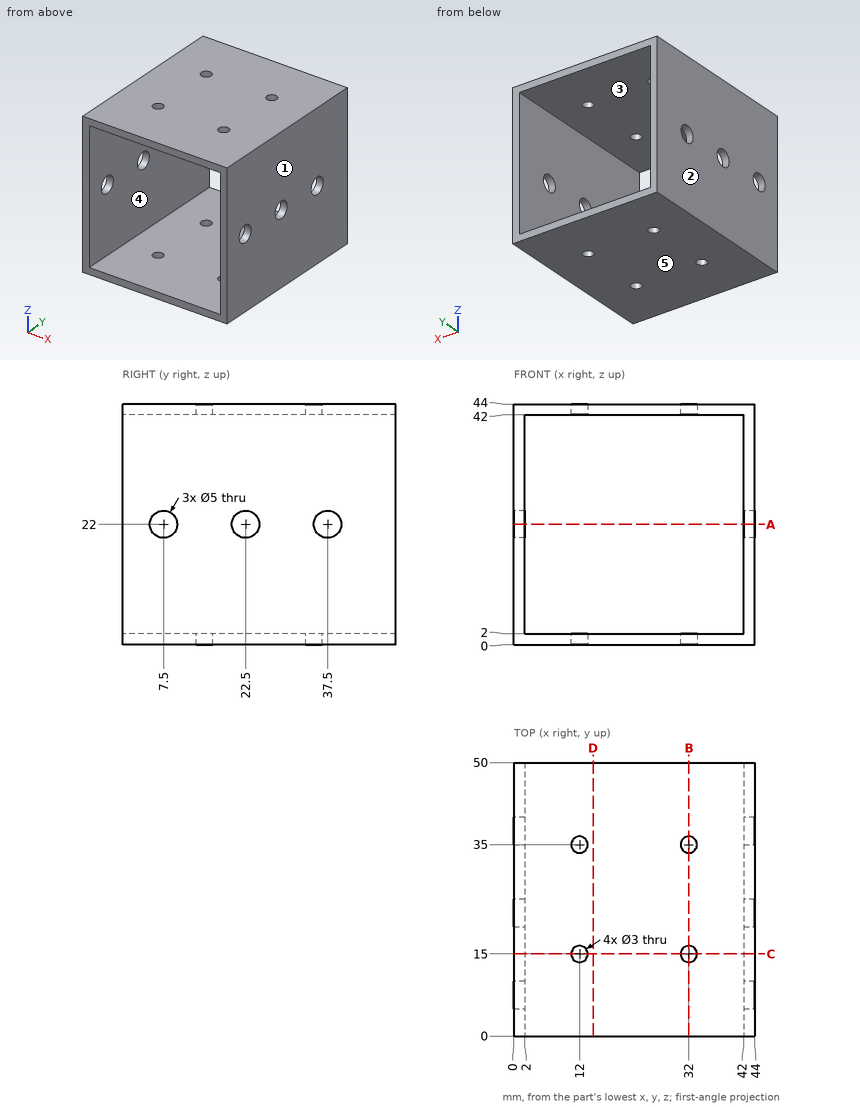
Geometry: see drawing. Coordinates: mm, zero at the bounding-box minimum. A direction names the side the tool comes from. Coordinates: 2 decimals unless noted, no trailing zeros. Loops run counter-clockwise (first coordinate to the right, second up) from the corner with the lowest first, then second, coordinate; pieces in that order, holes last. Notation, with made-up numbers: (17, 43.25) - (28, 43.25) arc R20 ccw to (28, 77.25) - close; hole circle Ø3 at (-14.75, 61). An arc over 180 degrees is marked (long way). Return JSON: item names as keys, results as strings.
Q1. Contact query for a flat-ended pin moving along its axis: P1, Ø3, axis at y = 7.5, z = 22, coming from the +X side. Output: stop coordinate, or through.
Results:
{"P1": "through"}
Q2. Section B-B, the plane x = 32. Return loops of the section in (y, z), plus the area to 3 significant figures.
Results:
{"outline": "(0, 0) - (13.5, 0) - (13.5, 2) - (0, 2) - close; (0, 42) - (13.5, 42) - (13.5, 44) - (0, 44) - close; (16.5, 0) - (33.5, 0) - (33.5, 2) - (16.5, 2) - close; (16.5, 42) - (33.5, 42) - (33.5, 44) - (16.5, 44) - close; (36.5, 0) - (50, 0) - (50, 2) - (36.5, 2) - close; (36.5, 42) - (50, 42) - (50, 44) - (36.5, 44) - close", "area": "176 mm2"}
Q3. Section A-A, the plane z = 22. Give the number of separate pieces and of enclosed holes in the cut face, plus the area to 3 significant figures.
Results:
{"separate pieces": "8", "enclosed holes": "0", "area": "140 mm2"}
Q4. Section D-D, the plane x = 14.5. Return loops of the section in (y, z).
Results:
{"outline": "(0, 0) - (50, 0) - (50, 2) - (0, 2) - close; (0, 42) - (50, 42) - (50, 44) - (0, 44) - close"}
Q5. Section C-C, the plane y = 15. Return loops of the section in (x, z), plus the area to 3 significant figures.
Results:
{"outline": "(0, 0) - (10.5, 0) - (10.5, 2) - (2, 2) - (2, 42) - (10.5, 42) - (10.5, 44) - (0, 44) - close; (13.5, 0) - (30.5, 0) - (30.5, 2) - (13.5, 2) - close; (13.5, 42) - (30.5, 42) - (30.5, 44) - (13.5, 44) - close; (33.5, 0) - (44, 0) - (44, 44) - (33.5, 44) - (33.5, 42) - (42, 42) - (42, 2) - (33.5, 2) - close", "area": "312 mm2"}
Q6. Mould query, pull axis X, two halves, no side actions, for the marked faces 1, 2 and 3. Classes: released by +X, released by -X, zero draft, split by the parting line, or undercut.
Results:
{"face 1": "released by +X", "face 2": "released by -X", "face 3": "undercut"}
Q7. Access query for the marked faces 4 and 5. Directions: +Z, -Z, +X, -X, +Y, -Y. A direction counts if a zero-diameter tool reaches every point of the face in a straight line with its end or side. Return the directions, or none.
Results:
{"face 4": "+Y, -Y", "face 5": "-Z, +X, -X, +Y, -Y"}
Q8. Material intervals for line 1 along Y through (x, z) = (12, 1); line 2 along Z through (x, y) = (16.5, 41), sorted ascending.
Results:
{"line 1": "0 to 13.5, 16.5 to 33.5, 36.5 to 50", "line 2": "0 to 2, 42 to 44"}
